The drawing under review shows one solid part. Ordinate dimensions are in mm from its lowest x, y, z. A direction names the side the tool comes from. Give positions to 0.01 mm unless a question says otherwise; leave off trailing zeros. Order: outer loops, then holes, each group sorted by start corner. A loop starts at its lowest first (then second) coordinate and runs counter-clockwise, first axis right, second up. Notation, with made-up numbers: (-27.5, 78.25) - (4.5, 78.25) arc R4 cw to (4.5, 83.25) - close; hole circle Ø6 at (13, 19). An arc over 180 degrees is marked (long way). Answer as a JSON object with one key per item and string values. Group by question number.
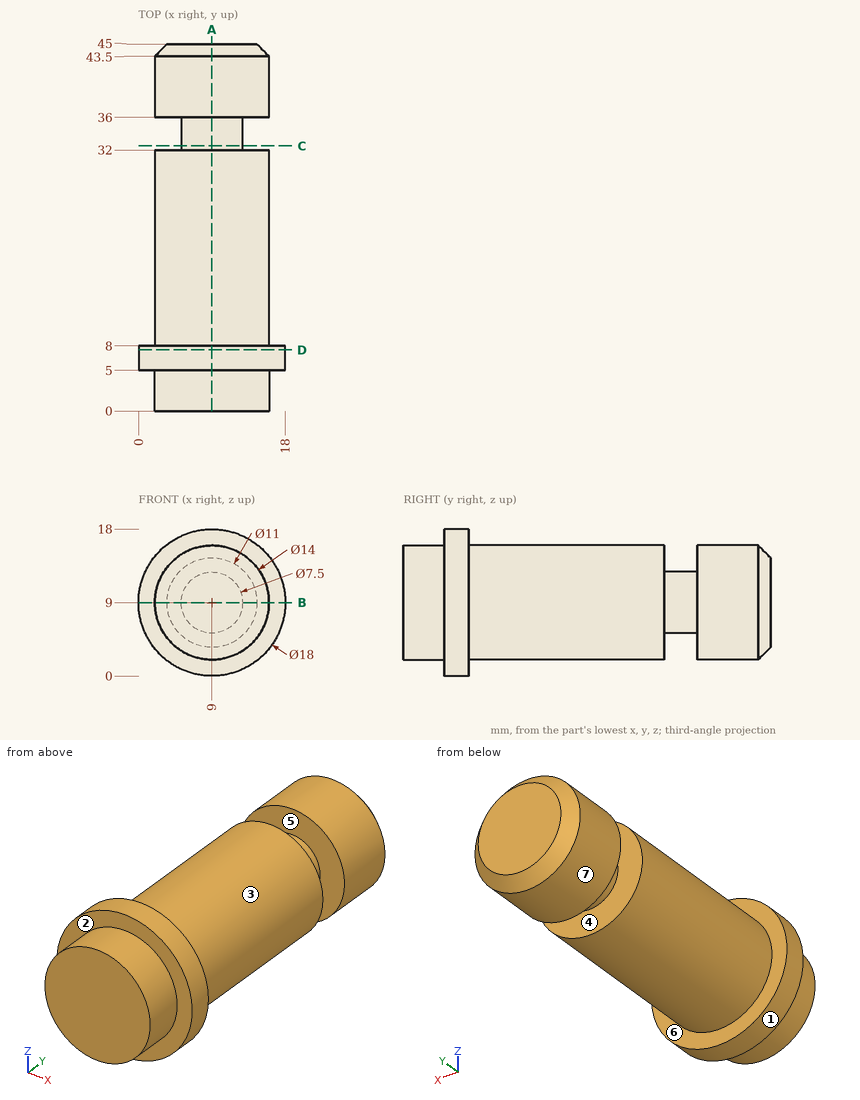
1) For the marked faces 1, 2 and 3, list the 3-axis set-ups (+Z, -Z, +X, -X, +Y, -Y) from which the entire face can be reached by the end or side of a thin tool; tool diameter is ignored.
2) For pin 1 (8 mm diameter, centred on x = 8, y = 39, fed in from -Z); pin 2 (5 mm diameter, centred on x = 15.5, y = 7.5, fed in from +Z); pin 3 (4 mm diameter, centred on x = 3, y = 13.5, fed in from +Z), all flat-tipped, find the tip position at first contact; note any pin that passes through.
3) Consider section D-D (y = 7.5). Give the boundary of the cut face in (x, z), plus the area to 3 significant figures.
4) Consider section C-C (y = 32.5). Give the boundary of the cut face in (x, z).
5) Consider section A-A (x = 9). Give the boundary of the cut face in (y, z), plus the area to 3 significant figures.
6) Consider section B-B (z = 9). Give the boundary of the cut face in (x, y), plus the area to 3 significant figures.
7) For line 1 (Y direction, x = 6, z = 13); line 2 (Y direction, x = 15.5, z = 11); line 3 (Y direction, x = 13.5, z = 3.5), list the stretches that pass through material, from the lowest coordinate up.
8) Mouldability with a two-part tool opening along Y and no side actions: class the marked faces 4, 5, 6 and 7 as released by +Y, released by -Y, zero draft, split by the parting line, or undercut.
Result set:
{
 "1": {"face 1": "+Y, -Y", "face 2": "-Y", "face 3": "+Y"},
 "2": {"pin 1": "stops at z = 2", "pin 2": "stops at z = 17.06", "pin 3": "stops at z = 14.74"},
 "3": {"outline": "circle Ø18 at (9, 9)", "area": "254 mm2"},
 "4": {"outline": "circle Ø7.5 at (9, 9)"},
 "5": {"outline": "(0, 2) - (5, 2) - (5, 0) - (8, 0) - (8, 2) - (32, 2) - (32, 5.25) - (36, 5.25) - (36, 2) - (43.5, 2) - (45, 3.5) - (45, 14.5) - (43.5, 16) - (36, 16) - (36, 12.75) - (32, 12.75) - (32, 16) - (8, 16) - (8, 18) - (5, 18) - (5, 16) - (0, 16) - close", "area": "614 mm2"},
 "6": {"outline": "(0, 5) - (2, 5) - (2, 0) - (16, 0) - (16, 5) - (18, 5) - (18, 8) - (16, 8) - (16, 32) - (12.75, 32) - (12.75, 36) - (16, 36) - (16, 43.5) - (14.5, 45) - (3.5, 45) - (2, 43.5) - (2, 36) - (5.25, 36) - (5.25, 32) - (2, 32) - (2, 8) - (0, 8) - close", "area": "614 mm2"},
 "7": {"line 1": "y = 0 to 32, 36 to 45", "line 2": "y = 0 to 32, 36 to 43.7", "line 3": "y = 5 to 8"},
 "8": {"face 4": "undercut", "face 5": "undercut", "face 6": "released by +Y", "face 7": "zero draft"}
}
